The figure shows three views and two pictorial views of one solid part (mm, origin at its lowest corner). Answer the questions. A direction names the side the tool comes from. Round coordinates to 2 decimals unless told otherwise and drop trailing zeros. Write each loop counter-clockwise with the first axis right and the second up, starting at its lowest first coordinate (ties: lowest second). Pieces come first, ordered by that corner, then holes. Notation, with made-up numbers: M -8.5,43.25 L 31.5,43.25 A29 cw 31.5,79.25 Z; hole C 63.5,-3.75 d9. An arc over 180 degrees is marked long. One line per item, written item: value. Start each with the question number.
Q1. Find section A-A (y = 20.5). Write down the section's boundary in (x, z).
Q2. Find section D-D (x = 12). Write down the section's boundary in (y, z).
Q3. A tool of negligible diameter and unlimited length cuts with its end or side. For the marked faces 1, 2 and 3, from which of +Z, -Z, +X, -X, +Y, -Y can it reach the whole face along a straight path? Write none if from no direction.
Q4. Consider probe 1 along Y at (x, z) = (2, 5.5); probe 2 along X at (y, z) = (14.5, 10); probe 3 along Y at (x, z) = (12.5, 9.5). Determine where each line is inside the solid, lowest interval first.
Q5. Find section C-C (z = 3). Write down the section's boundary in (x, y), and give its area (3 significant figures).
Q6. The mould has two halves that part along Z. Classify the marked faces 4, 5 and 6: released by +Z, released by -Z, zero draft, split by the parting line, or undercut.
Q7. Find section B-B (x = 2). Write down the section's boundary in (y, z).
Q8. Given pin 1 Ø1.3 at (x, z) = (2, 6) entering from -Y; pin 2 Ø1.5 at (y, z) = (31, 3.5) entering from +X; pin 3 Ø5 at (y, z) = (26, 7.5) entering from +X; pin 4 Ø3.5 at (x, y) = (30, 20.5) entering from +Z, each flat-ended and moving along its own axis, determine where each tip first touches the part or whether it passes through.
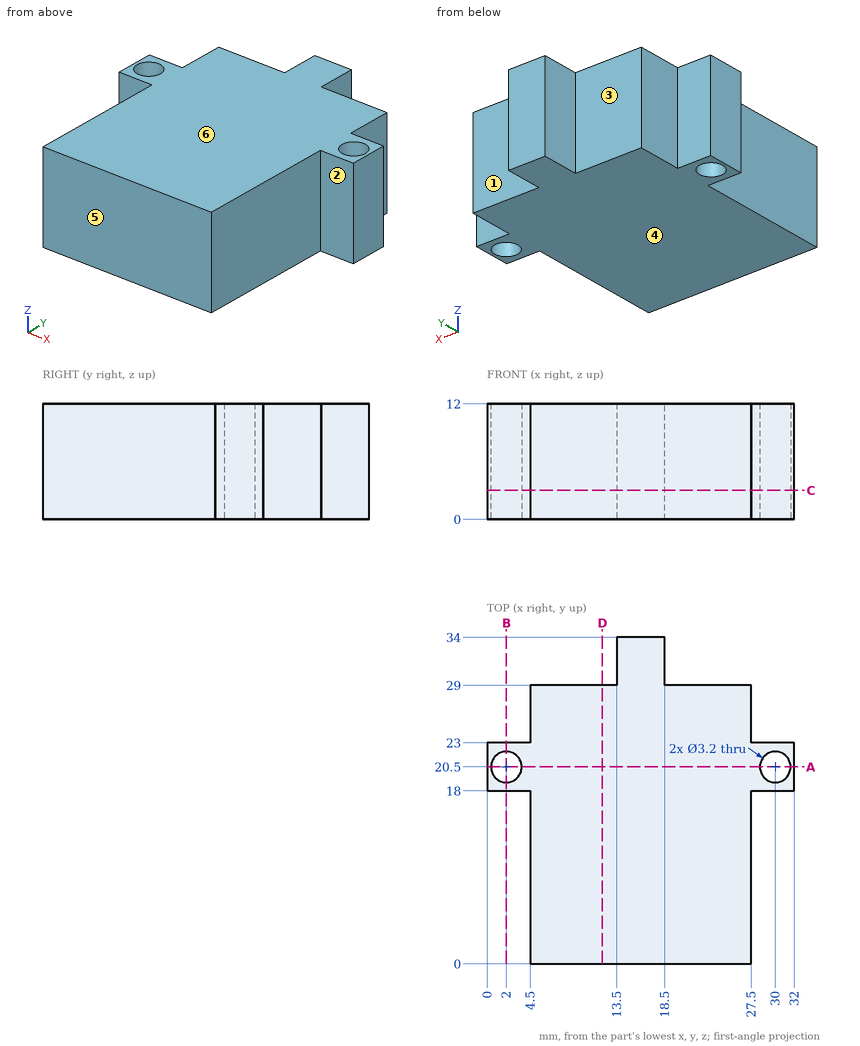
The answers:
1. outline: M 0,0 L 0.4,0 L 0.4,12 L 0,12 Z; M 3.6,0 L 28.4,0 L 28.4,12 L 3.6,12 Z; M 31.6,0 L 32,0 L 32,12 L 31.6,12 Z
2. outline: M 0,0 L 29,0 L 29,12 L 0,12 Z
3. face 1: +Z, -Z, +X, +Y
3. face 2: +Z, -Z, +X, -Y
3. face 3: +Z, -Z, -X, +Y
4. probe 1: 18 to 18.9, 22.1 to 23
4. probe 2: 4.5 to 27.5
4. probe 3: 0 to 29
5. outline: M 0,18 L 4.5,18 L 4.5,0 L 27.5,0 L 27.5,18 L 32,18 L 32,23 L 27.5,23 L 27.5,29 L 18.5,29 L 18.5,34 L 13.5,34 L 13.5,29 L 4.5,29 L 4.5,23 L 0,23 Z; hole C 2,20.5 d3.2; hole C 30,20.5 d3.2
5. area: 721 mm2
6. face 4: released by -Z
6. face 5: zero draft
6. face 6: released by +Z
7. outline: M 18,0 L 18.9,0 L 18.9,12 L 18,12 Z; M 22.1,0 L 23,0 L 23,12 L 22.1,12 Z
8. pin 1: y = 18
8. pin 2: x = 18.5
8. pin 3: x = 27.5
8. pin 4: z = 12
